Check sheet for the modelled part. Datum: model origin and axes. Units: mm. Face numbers are marked on the shaded views. A direction names the side the tool comes from. Give positions to 0.01 mm unless a question says otherwise; leave off trailing zeros. Order: outer loops, then holes, each group sorted by start corner. A loop starts at its lowest first (then second) coordinate and runs counter-clockwise, first axis right, second up.
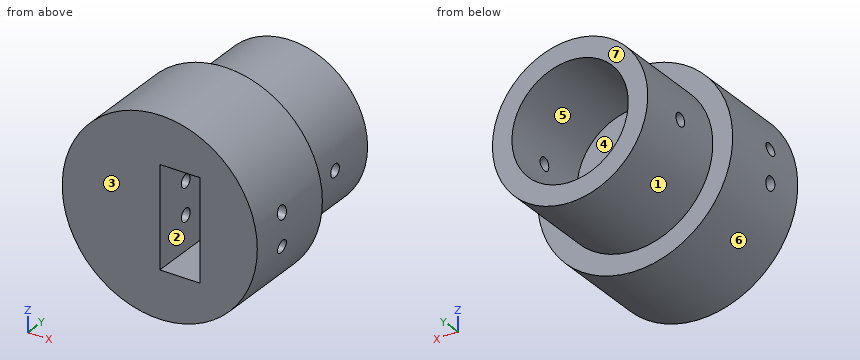
```python
from build123d import *

# Parameters (mm, degrees)
SKETCH1_R                = 15
BOSS_EXTRUDE1_DEPTH      = 15
SKETCH2_R                = 11.95
SKETCH2_R_2              = 8.95
BOSS_EXTRUDE2_DEPTH      = 15
BOSS_EXTRUDE2_DEPTH_BACK = 3
SKETCH3_R                = 1
CUT_EXTRUDE1_DEPTH       = 16
CUT_EXTRUDE1_DEPTH_BACK  = 16
SKETCH4_R                = 11
BOSS_EXTRUDE3_DEPTH      = 5
M3_CLEARANCE_HOLE1_D     = 3.4
SKETCH8_R                = 26.295997506
CUT_EXTRUDE2_DEPTH       = 66
SKETCH9_W                = 6.2
SKETCH9_H                = 15.5
CUT_EXTRUDE3_DEPTH       = 12


with BuildPart() as part:
    # Sketch1 → Boss-Extrude1 (new body)
    with BuildSketch(Plane(origin=(0, 0, 0), x_dir=(1, 0, 0), z_dir=(0, 1, 0))):
        Circle(SKETCH1_R)
    extrude(amount=BOSS_EXTRUDE1_DEPTH)

    # Sketch2 → Boss-Extrude2 (add, two sides)
    with BuildSketch(Plane(origin=(0, 15, 0), x_dir=(1, 0, 0), z_dir=(0, 1, 0))) as boss_extrude2_sk:
        Circle(SKETCH2_R)
        Circle(SKETCH2_R_2, mode=Mode.SUBTRACT)
    extrude(amount=BOSS_EXTRUDE2_DEPTH)
    extrude(boss_extrude2_sk.sketch, amount=-BOSS_EXTRUDE2_DEPTH_BACK)

    # Sketch3 → Cut-Extrude1 (cut, two sides)
    with BuildSketch(Plane(origin=(0, 0, 0), x_dir=(0, 0, -1), z_dir=(1, 0, 0))) as cut_extrude1_sk:
        with Locations((0, 22.5)):
            Circle(SKETCH3_R)
        with Locations((-2.5, 6)):
            Circle(SKETCH3_R)
        with Locations((2.5, 6)):
            Circle(SKETCH3_R)
    extrude(amount=CUT_EXTRUDE1_DEPTH, mode=Mode.SUBTRACT)
    extrude(cut_extrude1_sk.sketch, amount=-CUT_EXTRUDE1_DEPTH_BACK, mode=Mode.SUBTRACT)

    # Sketch4 → Boss-Extrude3 (add)
    with BuildSketch(Plane(origin=(0, 0, 0), x_dir=(0, 0, -1), z_dir=(1, 0, 0))):
        with BuildLine():
            Line((11, 0), (-11, 0))
            Line((-11, 0), (-11, -12))
            ThreePointArc((-11, -12), (-12.05572809, -16.472135955), (-15, -20))
            ThreePointArc((-15, -20), (0, -65), (15, -20))
            ThreePointArc((15, -20), (12.05572809, -16.472135955), (11, -12))
            Line((11, -12), (11, 0))
        make_face()
        with Locations((0, -40)):
            Circle(SKETCH4_R, mode=Mode.SUBTRACT)
    extrude(amount=BOSS_EXTRUDE3_DEPTH)

    # M3 Clearance Hole1 (through all)
    with Locations(Plane(origin=(5, 0, 0), x_dir=(0, 0, -1), z_dir=(1, 0, 0))):
        with Locations((10.606601718, -50.606601718), (-10.606601718, -50.606601718), (-10.606601718, -29.393398282), (10.606601718, -29.393398282)):
            Hole(M3_CLEARANCE_HOLE1_D / 2)

    # Sketch8 → Cut-Extrude2 (cut, through all)
    with BuildSketch(Plane.XZ):
        Circle(SKETCH8_R)
    extrude(amount=CUT_EXTRUDE2_DEPTH, mode=Mode.SUBTRACT)

    # Sketch9 → Cut-Extrude3 (cut)
    with BuildSketch(Plane.XZ):
        with Locations((3.1, 0)):
            Rectangle(SKETCH9_W, SKETCH9_H)
    extrude(amount=-CUT_EXTRUDE3_DEPTH, mode=Mode.SUBTRACT)


solid = part.part
```
(1) Cross-section at D-D on x = 10.5. Enter the section's corners in (y, z), then the cut area to 3 significant figures.
Response values:
outline: (0, -10.71) - (15, -10.71) - (15, -5.71) - (30, -5.71) - (30, 5.71) - (15, 5.71) - (15, 10.71) - (0, 10.71) - close; hole circle Ø2 at (6, -2.5); hole circle Ø2 at (6, 2.5); hole circle Ø2 at (22.5, 0)
area: 483 mm2
(2) Material ranges on L1, parallel to Y at x = 11.5, z = 2.5; L2, parallel to Z at x = 13.5, y = 6; L3, parallel to Y at x = 10, z = 0, recorded low to high.
Response values:
L1: y = 0 to 5, 7 to 30
L2: z = -6.54 to -3.5, -1.5 to 1.5, 3.5 to 6.54
L3: y = 0 to 21.5, 23.5 to 30
(3) Release check for a two-part mould opening along X. For the marked faces 4, 5, 6 and 7 record: released by +X, released by -X, zero draft, split by the parting line, or undercut.
Response values:
face 4: undercut
face 5: undercut
face 6: split by the parting line
face 7: zero draft
(4) Gauge pin test, flat ends, axial feed: pin 1 Ø1.5 at (x, y) = (8, 4) entering from +Z; pin 2 Ø2.5 at (y, z) = (22.5, 0) entering from -X; pin 3 Ø1.5 at (x, y) = (2.5, 17) entering from -Z; pin 4 Ø1.2 at (y, z) = (6, -2.5) entering from +X. Record the tip position at first contact, or that the pin passes through.
Response values:
pin 1: stops at z = 13.13
pin 2: stops at x = -11.95
pin 3: stops at z = -11.82
pin 4: passes through
(5) Cross-section at A-A on y = 3. Enter the section's corners in (x, z), then the cut area to 3 significant figures.
Response values:
outline: circle Ø30 at (0, 0); hole (0, -7.75) - (6.2, -7.75) - (6.2, 7.75) - (0, 7.75) - close
area: 611 mm2
(6) Set-up check for the marked faces 1, 2 and 3: record each of +Z, -Z, +X, -X, +Y, -Y from which the full face is reachable in a straight line by a thin tool's end or side.
Response values:
face 1: +Y
face 2: -Y
face 3: +Z, -Z, +X, -X, -Y
(7) Cross-section at B-B on z = 3. Enter the section's corners in (x, y).
Response values:
outline: (-14.7, 0) - (0, 0) - (0, 5.13) - (-14.7, 5.13) - close; (-14.7, 6.87) - (0, 6.87) - (0, 12) - (6.2, 12) - (6.2, 6.87) - (14.7, 6.87) - (14.7, 15) - (11.57, 15) - (11.57, 30) - (8.43, 30) - (8.43, 15) - (-8.43, 15) - (-8.43, 30) - (-11.57, 30) - (-11.57, 15) - (-14.7, 15) - close; (6.2, 0) - (14.7, 0) - (14.7, 5.13) - (6.2, 5.13) - close
